Geometry: see drawing. Coordinates: mm, zero at the bounding-box minimum. A direction names the side the tool comes from. Round coordinates to 2 decimals unless told otherwise and drop trailing zeros. Order: outer loops, then holes, each group sorted by start corner. A loop starts at its lowest first (then second) coordinate and runs counter-clockwise, first axis right, second up. Notation, with made-up numbers: (-32.5, 15) -> (-0.5, 15) arc R11 cw to (-0.5, 35) -> close; hole circle Ø9 at (80, -17.75). An arc over 180 degrees is marked (long way). Answer as CSV lines item,"result". Start each with the question number.
(1) Section query B-B (y = 6). Output: boundary loops of the cut face in (x, z) (3 decimals), plus the area to 3 significant figures.
(2) Line query: line 1 along Y through (x, z) = (27, 6.25) (3 decimals); line 2 along Y through (x, z) = (4, 13); line 3 along X through (y, z) = (38, 12) (3 decimals). Output: solid intervals per line, ascending. Write a range as from..to.
(3) Section query D-D (y = 38). Output: boundary loops of the cut face in (x, z) (3 decimals), plus the area to 3 significant figures.
(4) Set-up query: the marked faces 1, 2 and 3. Return all of +Z, -Z, +X, -X, +Y, -Y with unobstructed straight access to the full face (end or side cutting, diameter ignored); none if empty.
(5) Section query C-C (x = 27). Output: boundary loops of the cut face in (y, z) (3 decimals), plus the area to 3 significant figures.
(6) Pull-direction query (X, two-part tool) for the marked faces 4, 5, 6 and 7; classes: +X half, -X half, draft (parallel to the pull), parting line (faces both ways), or undercut.
(7) Section query A-A (z = 10). Output: boundary loops of the cut face in (x, y) (3 decimals).
(8) Contact query for flat-ended pins moving along their axis: P1, Ø3, axis at x = 15, z = 10, coming from the -Y side; P2, Ø1.2, axis at x = 2, y = 38, coming from the +Z side. Output: stop coordinate, or through.
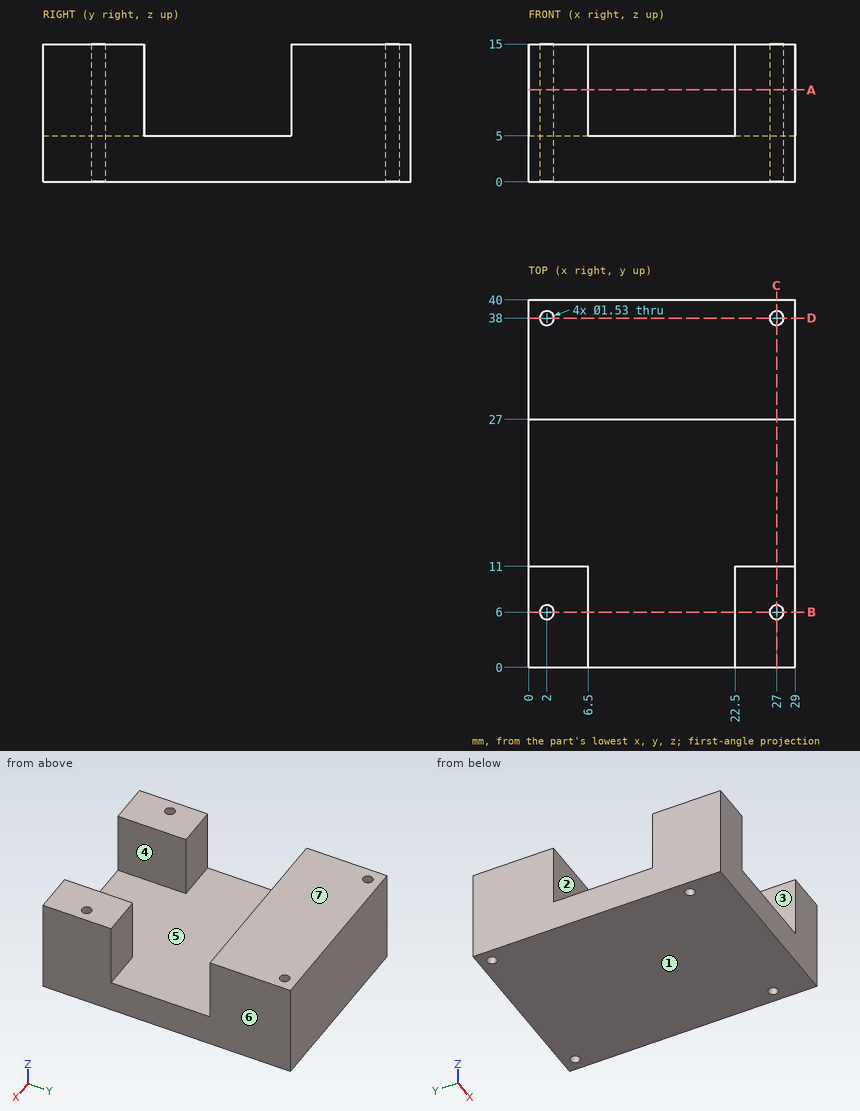
Answer block:
1,outline,"(0, 0) -> (1.235, 0) -> (1.235, 15) -> (0, 15) -> close; (2.765, 0) -> (26.235, 0) -> (26.235, 15) -> (22.5, 15) -> (22.5, 5) -> (6.5, 5) -> (6.5, 15) -> (2.765, 15) -> close; (27.765, 0) -> (29, 0) -> (29, 15) -> (27.765, 15) -> close"
1,area,"229 mm2"
2,line 1,"0..5.235, 6.765..11, 27..37.235, 38.765..40"
2,line 2,"0..11, 27..40"
2,line 3,"0..1.235, 2.765..26.235, 27.765..29"
3,outline,"(0, 0) -> (1.235, 0) -> (1.235, 15) -> (0, 15) -> close; (2.765, 0) -> (26.235, 0) -> (26.235, 15) -> (2.765, 15) -> close; (27.765, 0) -> (29, 0) -> (29, 15) -> (27.765, 15) -> close"
3,area,"389 mm2"
4,face 1,"-Z, +X, -X, +Y, -Y"
4,face 2,"+Z, +X, -X"
4,face 3,"+Z, -Y"
5,outline,"(0, 0) -> (5.235, 0) -> (5.235, 15) -> (0, 15) -> close; (6.765, 0) -> (37.235, 0) -> (37.235, 15) -> (27, 15) -> (27, 5) -> (11, 5) -> (11, 15) -> (6.765, 15) -> close; (38.765, 0) -> (40, 0) -> (40, 15) -> (38.765, 15) -> close"
5,area,"394 mm2"
6,face 4,"undercut"
6,face 5,"undercut"
6,face 6,"+X half"
6,face 7,"draft"
7,outline,"(0, 0) -> (6.5, 0) -> (6.5, 11) -> (0, 11) -> close; (0, 27) -> (29, 27) -> (29, 40) -> (0, 40) -> close; (22.5, 0) -> (29, 0) -> (29, 11) -> (22.5, 11) -> close; hole circle Ø1.53 at (2, 6); hole circle Ø1.53 at (2, 38); hole circle Ø1.53 at (27, 6); hole circle Ø1.53 at (27, 38)"
8,P1,"y = 27"
8,P2,"through"
